Input: part model. Units: mm. Frame: model coordinates. Face numbers are marked on the shaded views. Coordinates: 2 decimals unless noted, no trailing zeros. Order: outer loops, then holes, each group sorted by start corner. A loop starts at its lowest first (then second) coordinate and runs counter-clockwise, first axis right, second up. Notation, with made-up numbers: (54.5, 22.5) -> (66.5, 22.5) arc R31 cw to (66.5, 51.5) -> close; hole circle Ø10 at (41.25, -26). An arc over 180 degrees is marked (long way). Use one line per item in the form item = value. Start each with the question number.
1) Section query A-A on y = -16. Output: boundary loops of the cut face in (x, z) (3 decimals).
2) Pin query (flat end, axial travel): pin 1 (8 mm diameter, centred on x = 51.5, z = 25.5, fed in from +Y). Return the tip coordinate at first contact, or that it passes through.
3) Section query B-B on z = 23. Output: boundary loops of the cut face in (x, y), then the cut area to 3 significant figures.
4) Draft query along X for the marked faces 1, 2 and 3. Return one class per face: pulls with the +X half, pulls with the -X half, needs draft (parallel to the pull), parting line crosses it, or undercut.
5) Section query C-C on x = 40. Output: boundary loops of the cut face in (y, z), then the cut area to 3 significant figures.
6) Ray query, line 1 along Z through (x, y) = (49, -15.5); line 2 along Z through (x, y) = (44, -2); line 3 along X through (y, z) = (-2.25, 26). Return the intervals inside material, ascending.
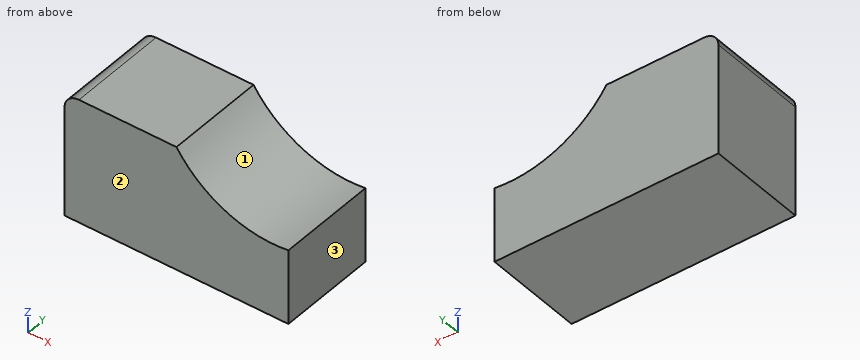
from build123d import *

# Parameters (mm, degrees)
F0_W     = 57.15
F0_H     = 31.75
F1_DEPTH = 25.4
F3_DEPTH = 25.4
F4_R     = 3.679261


with BuildPart() as f1:
    # F0 (on Front) → F1 (new body)
    with BuildSketch(Plane.XZ):
        with Locations((28.575, 15.875)):
            Rectangle(F0_W, F0_H)
    extrude(amount=F1_DEPTH)

    # F2 (on face) → F3 (cut)
    with BuildSketch(Plane.XZ.offset(25.4)):
        with BuildLine():
            Line((57.15, 31.75), (28.575, 31.75))
            ThreePointArc((28.575, 31.75), (41.05591, 21.335173), (57.15, 19.05))
            Line((57.15, 19.05), (57.15, 31.75))
        make_face()
    extrude(amount=-F3_DEPTH, mode=Mode.SUBTRACT)

    # F4
    f4_edges = [f1.edges().sort_by_distance(p)[0] for p in [
        (0, -12.7, 31.75),
    ]]
    fillet(f4_edges, radius=F4_R)


solid = f1.part
Answers below:
q1.outline = (0, 0) -> (57.15, 0) -> (57.15, 19.05) arc R29.702 cw to (28.575, 31.75) -> (3.679, 31.75) arc R3.679 ccw to (0, 28.071) -> close
q2.pin_1 = through
q3.outline = (0, -25.4) -> (37.85, -25.4) -> (37.85, 0) -> (0, 0) -> close
q3.area = 961 mm^2
q4.face_1 = undercut
q4.face_2 = needs draft
q4.face_3 = pulls with the +X half
q5.outline = (-25.4, 0) -> (0, 0) -> (0, 21.83) -> (-25.4, 21.83) -> close
q5.area = 554 mm^2
q6.line_1 = 0 to 19.06
q6.line_2 = 0 to 20.21
q6.line_3 = 0 to 33.7
